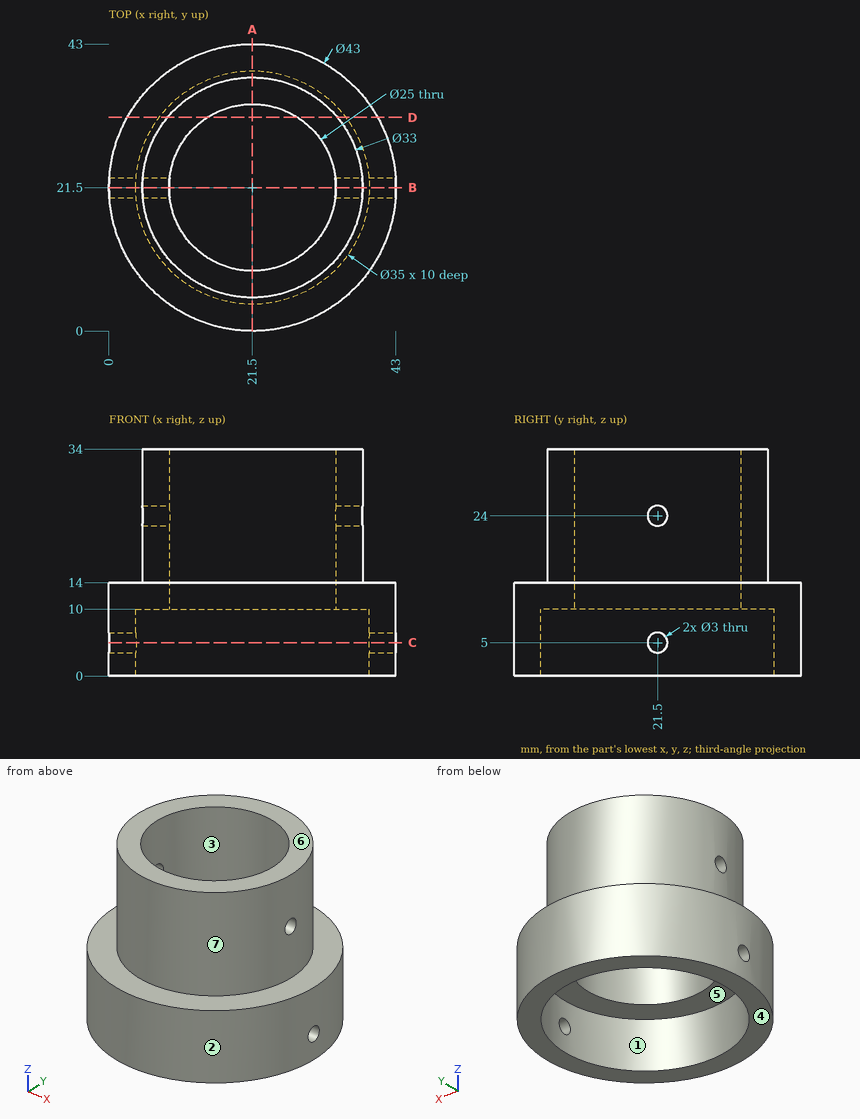
Part print with two shaded views. Sizes in mm from the minimum x, y, z corner. A direction names the side the tool comes from. Round coordinates to 2 decimals unless told otherwise and drop trailing zeros. Order: outer loops, then holes, each group sorted by start corner. A loop starts at its lowest first (then second) coordinate and runs counter-clockwise, first axis right, second up. Notation, with made-up numbers: M -34,-38 L 9,-38 A21 ccw 9,-24 Z; hole C 60.5,31.5 d1. An arc over 180 degrees is marked long. Answer in a Markdown table with one row per item. Add a question column.
Q1. 3-axis set-ups, long thin cutter, end or side, ignore diameter. For the marked faces 5, 6 and 7: which of +Z, -Z, +X, -X, +Y, -Y reach the whole face in a straight line?
Q2. Cut at A-A on x = 21.5. Give the cut face in (y, z).
Q3. Cut at B-B on y = 21.5. Give the number of separate pieces and of enclosed holes in the cut face, and give its area (3 significant figures).
Q4. Cut at D-D on y = 32. Give the cut face in (x, z), and give its area (3 significant figures).
Q5. Cut at C-C on z = 5. Give the cut face in (x, y), and give its area (3 significant figures).
Q6. Pin check, flat tips, straight feed: pin 1 (5 mm diameter, centred on y = 35, z = 27, fed in from -X); pin 2 (4 mm diameter, centred on y = 37, z = 29, fed in from +X); pin 3 (1 mm diameter, centred on y = 29, z = 27.5, fed in from +X); pin 4 (3.5 mm diameter, centred on y = 21.5, z = 5, fed in from +X). Stop position of each tip, or through.
Q7. Mould opens along Y. For the marked faces 1, 2, 3 and 4 say: +Y half, -Y half, draft (parallel to the pull), parting line (faces both ways), or undercut.
Q8. Wall check: L1, parallel to X at y = 22, z = 32; L2, parallel to Y at x = 21.5, z = 5.5. Give the ranges that are in metal, low to high. Write a range as from..to.
Established:
| question | item | result |
|---|---|---|
| 1 | face 5 | -Z |
| 1 | face 6 | +Z, +X, -X, +Y, -Y |
| 1 | face 7 | +Z |
| 2 | outline | M 0,0 L 4,0 L 4,10 L 9,10 L 9,34 L 5,34 L 5,14 L 0,14 Z; M 34,10 L 39,10 L 39,0 L 43,0 L 43,14 L 38,14 L 38,34 L 34,34 Z |
| 3 | separate pieces | 6 |
| 3 | enclosed holes | 0 |
| 3 | area | 264 mm2 |
| 4 | outline | M 2.74,0 L 7.5,0 L 7.5,10 L 14.72,10 L 14.72,34 L 8.77,34 L 8.77,14 L 2.74,14 Z; M 28.28,10 L 35.5,10 L 35.5,0 L 40.26,0 L 40.26,14 L 34.23,14 L 34.23,34 L 28.28,34 Z |
| 4 | area | 429 mm2 |
| 5 | outline | M 0.05,20 A21.5 ccw 42.95,20 L 38.94,20 A17.5 cw 4.06,20 Z; M 0.05,23 L 4.06,23 A17.5 cw 38.94,23 L 42.95,23 A21.5 ccw Z |
| 5 | area | 466 mm2 |
| 6 | pin 1 | stops at x = 9.2 |
| 6 | pin 2 | stops at x = 30.99 |
| 6 | pin 3 | stops at x = 36.44 |
| 6 | pin 4 | stops at x = 43 |
| 7 | face 1 | undercut |
| 7 | face 2 | parting line |
| 7 | face 3 | undercut |
| 7 | face 4 | draft |
| 8 | L1 | x = 5.01..9.01, 33.99..37.99 |
| 8 | L2 | y = 0..4, 39..43 |
